Here's how the part is built. I have some questions about the finished solid (model axes, mm). Round coordinates to 2 decimals unless told otherwise and drop trailing zeros. Write each loop counter-clockwise with the first axis right and the second up, starting at its lowest first coordinate (ties: lowest second). Pieces come first, ordered by that corner, then holes. Notation, with made-up numbers: (67.5, 69) -> (99.5, 69) arc R21 cw to (99.5, 73) -> close; hole circle Ø8 at (-9, 88). An arc over 180 degrees is marked (long way). Put each result on its own line as item: value. Start each with the question number.
1) Will these pins go through, and if not, where does the flat tip stop? P1, Ø1.5, axis at y = 1, z = 44, coming from the -X side; P2, Ø3, axis at y = 3.5, z = 29.5, coming from the -X side; P3, Ø2, axis at x = 1.5, z = 26.5, coming from the +Y side; P4, Ø3.5, axis at x = 0, z = 5, coming from the -Y side.
2) I want a section at C-C, the plane y = -2.5. List the corners of the cut face in (x, z) for me, then the cut area to 3 significant figures.
3) I want a section at A-A, the plane x = 0. List the corners of the cut face in (y, z) for me, then the cut area to 3 significant figures.
4) If I drill on line 1 along Z through (x, y) = (1.75, 0.5); line 2 along Z through (x, y) = (1, -0.5); line 3 along X through (y, z) = (0.5, 5), over which ranges is the centre line in solid material (lowest first)? Write a range as [from, to].
5) I want a section at D-D, the plane z = 48. List the corners of the cut face in (x, y) for me.
6) I want a section at B-B, the plane z = 5. List the corners of the cut face in (x, y) for me.
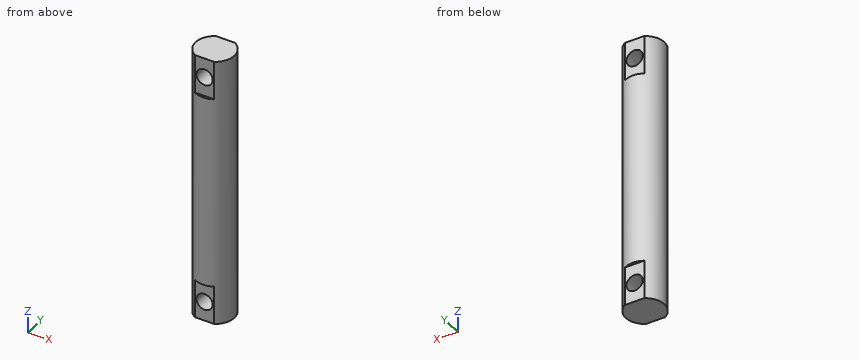
from build123d import *

# Parameters (mm, degrees)
SKETCH_1_R          = 5
EXTRUDE_1_DEPTH     = 70
SKETCH_2_R          = 2.1
CUT_EXTRUDE_1_DEPTH = 5
SKETCH_3_W          = 5
SKETCH_3_H          = 10
CUT_EXTRUDE_2_DEPTH = 10
SKETCH_4_W          = 5
SKETCH_4_H          = 10
CUT_EXTRUDE_3_DEPTH = 10


with BuildPart() as part:
    # 草图1 → 凸台-拉伸1 (new body)
    with BuildSketch(Plane.XY):
        Circle(SKETCH_1_R)
    extrude(amount=EXTRUDE_1_DEPTH)

    # 草图2 → 切除-拉伸1 (cut, symmetric)
    with BuildSketch(Plane(origin=(0, 0, 0), x_dir=(1, 0, 0), z_dir=(0, 1, 0))):
        with Locations(Location((0, -5, 0), (0, 0, 270))):
            Circle(SKETCH_2_R)
        with Locations(Location((0, -65, 0), (0, 0, 270))):
            Circle(SKETCH_2_R)
    extrude(amount=CUT_EXTRUDE_1_DEPTH, both=True, mode=Mode.SUBTRACT)

    # 草图3 → 切除-拉伸2 (cut)
    with BuildSketch(Plane.XY.offset(70)):
        with Locations((0, 9.330127019)):
            Rectangle(SKETCH_3_W, SKETCH_3_H)
        with Locations((0, -9.330127019)):
            Rectangle(SKETCH_3_W, SKETCH_3_H)
    extrude(amount=-CUT_EXTRUDE_2_DEPTH, mode=Mode.SUBTRACT)

    # 草图4 → 切除-拉伸3 (cut)
    with BuildSketch(Plane(origin=(0, 0, 0), x_dir=(-1, 0, 0), z_dir=(0, 0, -1))):
        with Locations((0, 9.330127019)):
            Rectangle(SKETCH_4_W, SKETCH_4_H)
        with Locations((0, -9.330127019)):
            Rectangle(SKETCH_4_W, SKETCH_4_H)
    extrude(amount=-CUT_EXTRUDE_3_DEPTH, mode=Mode.SUBTRACT)


solid = part.part
Findings:
1. P1: stops at x = -4.99
1. P2: stops at x = -4.58
1. P3: stops at y = 4.97
1. P4: passes through
2. outline: (-4.33, 0) -> (4.33, 0) -> (4.33, 70) -> (-4.33, 70) -> close; hole circle Ø4.2 at (0, 5); hole circle Ø4.2 at (0, 65)
2. area: 579 mm2
3. outline: (-5, 10) -> (-4.33, 10) -> (-4.33, 7.1) -> (4.33, 7.1) -> (4.33, 10) -> (5, 10) -> (5, 60) -> (4.33, 60) -> (4.33, 62.9) -> (-4.33, 62.9) -> (-4.33, 60) -> (-5, 60) -> close; (-4.33, 0) -> (4.33, 0) -> (4.33, 2.9) -> (-4.33, 2.9) -> close; (-4.33, 67.1) -> (4.33, 67.1) -> (4.33, 70) -> (-4.33, 70) -> close
3. area: 600 mm2
4. line 1: z = [0, 3.84], [6.16, 63.84], [66.16, 70]
4. line 2: z = [0, 3.15], [6.85, 63.15], [66.85, 70]
4. line 3: x = [-4.97, -2.1], [2.1, 4.97]
5. outline: circle Ø10 at (0, 0)
6. outline: (-2.5, -4.33) -> (-2.1, -4.33) -> (-2.1, 4.33) -> (-2.5, 4.33) arc R5 ccw to start; (2.1, -4.33) -> (2.5, -4.33) arc R5 ccw to (2.5, 4.33) -> (2.1, 4.33) -> close
